The figure shows three views and two pictorial views of one solid part (mm, origin at its lowest corner). Answer the questions. A direction names the side the tool comes from. Give positions to 0.01 mm unless a question says otherwise; leave off trailing zeros. Order: outer loops, then holes, each group sorted by start corner. A loop starts at its lowest first (then second) coordinate and runs counter-clockwise, first axis right, second up. Notation, with made-up numbers: (-11, 26.5) -> (-4, 26.5) arc R18 ccw to (-4, 44.5) -> close; hole circle Ø4 at (27.25, -19). An arc over 180 degrees is marked (long way). Use one line per item in the form item = value.
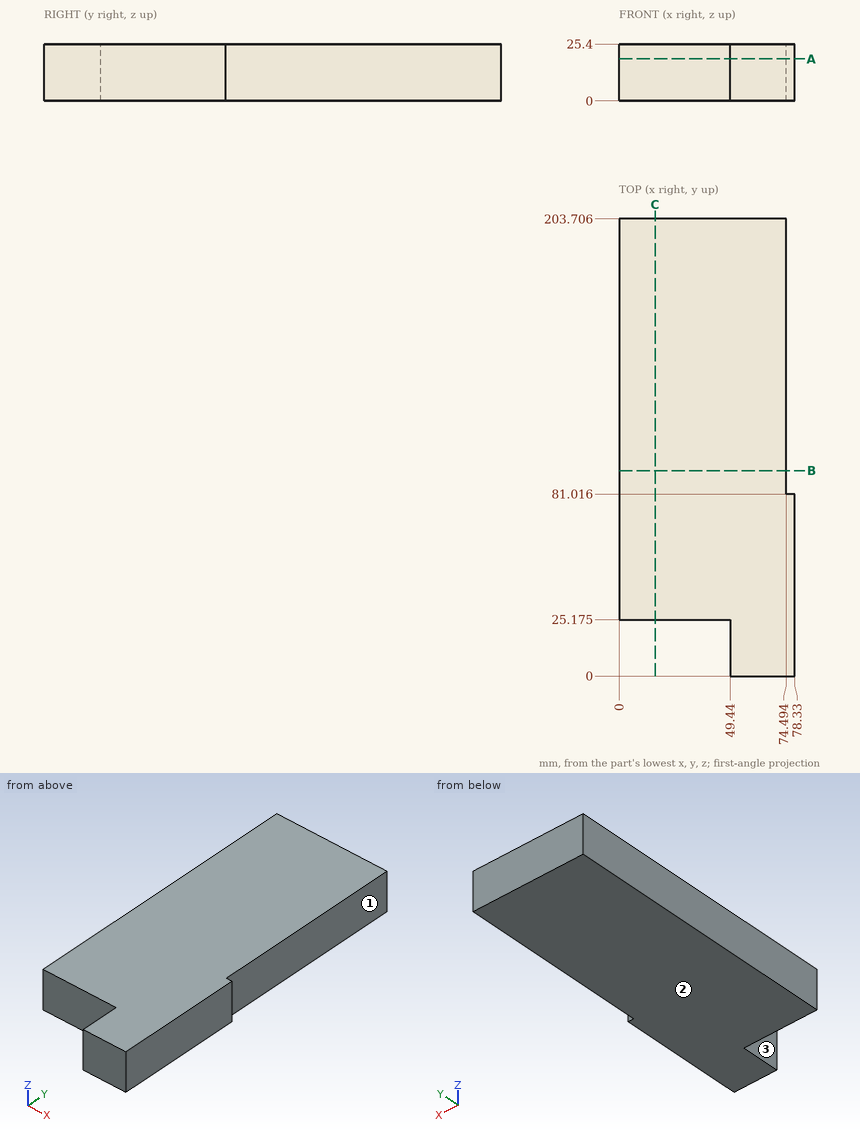
Item 1: Straight lines are drawn through the part: L1, parallel to X at y = 84.5, z = 12.25; L2, parallel to Y at x = 27.5, z = 2 (1 decimal); L3, parallel to X at y = 22.5, z = 12.25. For each, find the intervals that lie inside material, in ascending order. Write a range as from..to.
Checks:
L1 = 0..74.49
L2 = 25.2..203.7
L3 = 49.44..78.33
Item 2: The part is cut by section C-C on x = 16. Give the vertices of the cut face in (y, z) (1 decimal).
Checks:
outline = (25.2, 0) -> (203.7, 0) -> (203.7, 25.4) -> (25.2, 25.4) -> close
Item 3: The part is cut by section A-A on z = 18.75. Give the vertices of the cut face in (x, y) (1 decimal), and give its area (3 significant figures).
Checks:
outline = (0, 25.2) -> (49.4, 25.2) -> (49.4, 0) -> (78.3, 0) -> (78.3, 81) -> (74.5, 81) -> (74.5, 203.7) -> (0, 203.7) -> close
area = 14,200 mm²
Item 4: The part is cut by section B-B on y = 91.5. Give the vertices of the cut face in (x, z).
Checks:
outline = (0, 0) -> (74.49, 0) -> (74.49, 25.4) -> (0, 25.4) -> close
Item 5: Which of the six approach directions +Z, -Z, +X, -X, +Y, -Y give full straight-line access (tool end or side, diameter ignored) to the marked faces 1, 2 and 3?
Checks:
face_1 = +Z, -Z, +X, +Y
face_2 = -Z, +X, -X, +Y, -Y
face_3 = +Z, -Z, -X, -Y
Item 6: Given pin 1 Ø8 at (x, z) = (28.5, 5.5) entering from -Y (3 decimals); pin 2 Ø3 at (x, z) = (77, 11.5) entering from +Y; pin 3 Ø4 at (y, z) = (84, 21.5) entering from +X, each flat-ended and moving along its own axis, determine where each tip first touches the part or whether it passes through.
Checks:
pin_1 = 25.175
pin_2 = 81.02
pin_3 = 74.49
